from build123d import *

# Parameters (mm, degrees)
F1_DEPTH = 6
F2_W     = 20
F2_H     = 5.42
F3_DEPTH = 2
F4_R     = 2.25
F5_DEPTH = 8.001
F6_R     = 3.75
F7_DEPTH = 2
F8_SIZE  = 3


with BuildPart() as f1:
    # F0 (on Top) → F1 (new body)
    with BuildSketch(Plane.XY):
        Polygon((-30, 0), (-10, 0), (-10, -20), (0, -20), (10, -20), (10, 0), (30, 0), (30, 20), (0, 20), (-30, 20), align=None)
    extrude(amount=F1_DEPTH)

    # F2 (on face) → F3 (join)
    with BuildSketch(Plane.XY.offset(6)):
        Polygon((2.71, 0), (0, 0), (-2.71, 0), (-2.71, -20), (2.71, -20), align=None)
        Polygon((7.845558, 12.71), (7.845558, 10), (7.845558, 7.29), (30, 7.29), (30, 12.71), align=None)
        with Locations((-20, 10)):
            Rectangle(F2_W, F2_H)
    extrude(amount=F3_DEPTH)

    # F4 (on face) → F5 (cut, through all)
    with BuildSketch(Plane(origin=(0, 0, 0), x_dir=(1, 0, 0), z_dir=(0, 0, -1))):
        with Locations((-20, -10)):
            Circle(F4_R)
        with Locations((0, -10)):
            Circle(F4_R)
        with Locations((0, 10)):
            Circle(F4_R)
        with Locations((20.741304, -10)):
            Circle(F4_R)
    extrude(amount=-F5_DEPTH, mode=Mode.SUBTRACT)

    # F6 (on face) → F7 (cut)
    with BuildSketch(Plane(origin=(0, 0, 0), x_dir=(1, 0, 0), z_dir=(0, 0, -1))):
        with Locations((0, 10)):
            Circle(F6_R)
        with Locations((0, -10)):
            Circle(F6_R)
        with Locations((20.741304, -10)):
            Circle(F6_R)
        with Locations((-20, -10)):
            Circle(F6_R)
    extrude(amount=-F7_DEPTH, mode=Mode.SUBTRACT)

    # F8
    f8_edges = [f1.edges().sort_by_distance(p)[0] for p in [
        (-10, -10, 0),
        (-20, 0, 0),
        (10, -10, 0),
        (20, 0, 0),
        (0, 20, 0),
        (30, 10, 0),
        (-30, 10, 0),
        (0, -20, 0),
    ]]
    chamfer(f8_edges, length=F8_SIZE)


solid = f1.part
Read the model definition and answer for the solid it produces. Units are mm, in the model's axes. A direction names the side the tool comes from. Give positions to 0.01 mm unless a question says otherwise; leave off trailing zeros. Loops run counter-clockwise (first coordinate to the right, second up) from the corner with the lowest first, then second, coordinate; pieces in that order, holes last. Notation, with made-up numbers: (67, 22.5) - (95, 22.5) arc R21 cw to (95, 47.5) - close; hole circle Ø11 at (46.25, 43.25). An arc over 180 degrees is marked (long way). Answer as CSV lines item,"result". Start each with the question number.
1) Find section C-C (x = 0). Write down the section's boundary in (y, z), then the cut area to 3 significant figures.
2) Find section B-B (z = 4). Write down the section's boundary in (x, y).
3) Find section A-A (y = 10). State how many separate pieces and enclosed holes the cut face has, then the cut area to 3 significant figures.
4) Which of the six approach directions +Z, -Z, +X, -X, +Y, -Y give full straight-line access (tool end or side, diameter ignored) to faces 4 (the face through (10, -10, 4)), 5 (the face through (18, 1, 2)), 6 (the face through (-20, 0, 4)), 7 (the face through (-18, 12, 2))?
5) Each of these flat-tipped pins is pushed along its axis until it touches: pin 1 Ø1.5 at (x, z) = (-20, 3) entering from -Y; pin 2 Ø2.5 at (y, z) = (-7.5, 4.5) entering from -X; pin 3 Ø3 at (y, z) = (-8, 1) entering from +X. Where does it stop, or does it pass through?
6) Find section D-D (y = -1.5). Write down the section's boundary in (x, z).
7) Determine the mould class of faces 1 (the face through (-10, -10, 4)), 2 (the face through (19, 12.71, 7)), 3 (the face through (-0.488, 6.282, 0.986)) for opening direction Y: released by +Y, released by -Y, zero draft, split by the parting line, or undercut.
8) Straight lines are drawn through the part: L1, parallel to X at y = 10, z = 3.1; L2, parallel to Y at x = -20, z = 3.2; L3, parallel to X at y = 11, z = 2.5. For each, find the intervals that lie inside material, in ascending order. Write a range as from..to.
Findings below:
1,outline,"(-20, 3) - (-17, 0) - (-13.75, 0) - (-13.75, 2) - (-12.25, 2) - (-12.25, 8) - (-20, 8) - close; (-7.75, 2) - (-6.25, 2) - (-6.25, 0) - (6.25, 0) - (6.25, 2) - (7.75, 2) - (7.75, 6) - (0, 6) - (0, 8) - (-7.75, 8) - close; (12.25, 2) - (13.75, 2) - (13.75, 0) - (17, 0) - (20, 3) - (20, 6) - (12.25, 6) - close"
1,area,"196 mm^2"
2,outline,"(-30, 0) - (-10, 0) - (-10, -20) - (10, -20) - (10, 0) - (30, 0) - (30, 20) - (-30, 20) - close; hole circle Ø4.5 at (-20, 10); hole circle Ø4.5 at (0, -10); hole circle Ø4.5 at (0, 10); hole circle Ø4.5 at (20.74, 10)"
3,separate pieces,"4"
3,enclosed holes,"0"
3,area,"318 mm^2"
4,face 4,"+Z, -Z, +X, -Y"
4,face 5,"-Z, +X, -Y"
4,face 6,"+Z, -Z, -X, -Y"
4,face 7,"-Z"
5,pin 1,"y = 0"
5,pin 2,"x = -10"
5,pin 3,"x = 9.5"
6,outline,"(-10, 3) - (-7, 0) - (7, 0) - (10, 3) - (10, 6) - (2.71, 6) - (2.71, 8) - (-2.71, 8) - (-2.71, 6) - (-10, 6) - close"
7,face 1,"zero draft"
7,face 2,"released by +Y"
7,face 3,"undercut"
8,L1,"-30..-22.25, -17.75..-2.25, 2.25..18.49, 22.99..30"
8,L2,"0..7.75, 12.25..20"
8,L3,"-29.5..-22.02, -17.98..-2.02, 2.02..18.73, 22.76..29.5"
